```python
from build123d import *

# Parameters (mm, degrees)
SKETCH1_W           = 11
SKETCH1_H           = 22
BOSS_EXTRUDE1_DEPTH = 27
BOSS_EXTRUDE2_START = -8
SKETCH2_W           = 11
SKETCH2_H           = 5
BOSS_EXTRUDE2_DEPTH = 2


with BuildPart() as part:
    # Sketch1 → Boss-Extrude1 (new body)
    with BuildSketch(Plane(origin=(0, 0, 0), x_dir=(1, 0, 0), z_dir=(0, 1, 0))):
        with Locations((5.5, 11)):
            Rectangle(SKETCH1_W, SKETCH1_H)
    extrude(amount=BOSS_EXTRUDE1_DEPTH)

    # Sketch2 → Boss-Extrude2 (add)
    with BuildSketch(Plane.XZ.offset(BOSS_EXTRUDE2_START)):
        with Locations((5.5, 2.5)):
            Rectangle(SKETCH2_W, SKETCH2_H)
        with Locations((5.5, -24.5)):
            Rectangle(SKETCH2_W, SKETCH2_H)
    extrude(amount=-BOSS_EXTRUDE2_DEPTH)


solid = part.part
```
Model file for the job. Use its own axes, mm. A direction names the side the tool comes from. Coordinates: 2 decimals unless noted, no trailing zeros. Loops run counter-clockwise (first coordinate to the right, second up) from the corner with the lowest first, then second, coordinate; pieces in that order, holes last. Notation, with made-up numbers: M 67,59 L 97,59 A22 cw 97,69 Z; hole C 23,4 d7. An arc over 180 degrees is marked long. Use CSV: the item, a comma, the result in double quotes. Start each with the question number.
1. Band-saw the part on B-B, the plane y = 6.25. List the corners of the cut face in (x, z).
2. Probe probe 1 along Z at (x, y) = (7.75, 4.5); probe 2 along Y at (x, z) = (3.25, -24). List the from-to ranges inside material, lowest first. Write a range as [from, to].
3. Tool access for faces 1 (the flat face through (5, 4, 0)), 2 (the flat face through (5, 4, -22)), 3 (the flat face through (5, 18, -22)), 4 (the flat face through (5, 18, 0)), 5 (the flat face through (5, 9, 5)): list every direction of +Z, -Z, +X, -X, +Y, -Y with a clear straight run to the whole face (end or side of a thin tool).
4. Flat gauge pins, fed straight in: pin 1 (4 mm diameter, centred on x = 4.5, y = 24, fed in from +Z); pin 2 (1.5 mm diameter, centred on x = 3.5, z = -25, fed in from +Y); pin 3 (1.5 mm diameter, centred on x = 4.5, z = -23.5, fed in from -Y). Where does each tip first touch, or does it go through?
5. Band-saw the part on A-A, the plane x = 1.5. List the corners of the cut face in (y, z), then the cut area to 3 significant figures.
6. Band-saw the part on C-C, the plane z = 1. List the corners of the cut face in (x, y).
Entries:
1,outline,"M 0,-22 L 11,-22 L 11,0 L 0,0 Z"
2,probe 1,"z = [-22, 0]"
2,probe 2,"y = [8, 10]"
3,face 1,"+Z, +X, -X, -Y"
3,face 2,"-Z, +X, -X, -Y"
3,face 3,"-Z, +X, -X, +Y"
3,face 4,"+Z, +X, -X, +Y"
3,face 5,"+Z, +X, -X, +Y, -Y"
4,pin 1,"stops at z = 0"
4,pin 2,"stops at y = 10"
4,pin 3,"stops at y = 8"
5,outline,"M 0,-22 L 8,-22 L 8,-27 L 10,-27 L 10,-22 L 27,-22 L 27,0 L 10,0 L 10,5 L 8,5 L 8,0 L 0,0 Z"
5,area,"614 mm2"
6,outline,"M 0,8 L 11,8 L 11,10 L 0,10 Z"
